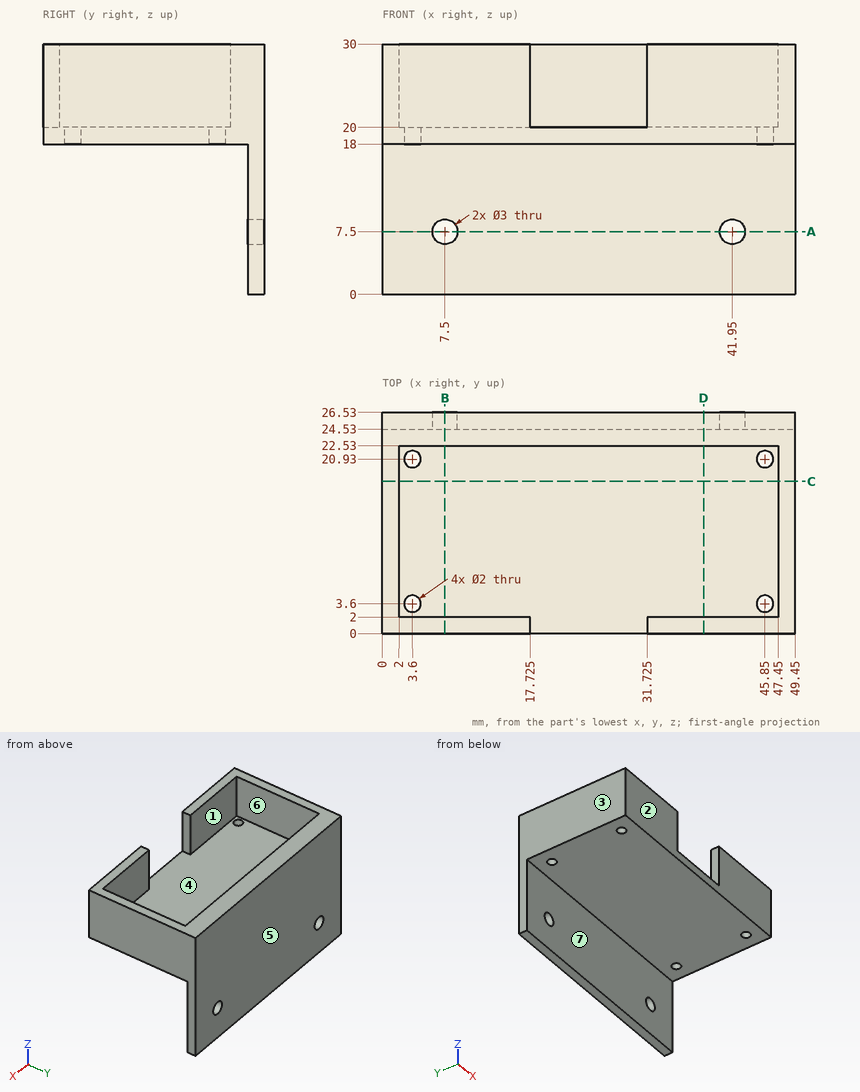
Could you check a few things on this drawing? It's one solid part, dimensions in mm from its lowest x, y, z. A direction names the side the tool comes from. Round coordinates to 2 decimals unless told otherwise and drop trailing zeros. Loops run counter-clockwise (first coordinate to the right, second up) from the corner with the lowest first, then second, coordinate; pieces in that order, holes last.
Q1. I want a section at D-D (x = 38.5). Write out the boundary of the cut face in (y, z).
Q2. On a 3-axis mill with a long thin cutter (end or side, diameter ignored), from which of +Z, -Z, +X, -X, +Y, -Y can I reach the whole of each face in a straight line? I mean the marked faces 5, 6 and 7. Say none if no direction works.
Q3. Please list where these lines run through material, in increasing order: L1, parallel to Y at x = 45.85, z = 18.5; L2, parallel to Y at x = 46, z = 25; L3, parallel to X at y = 14.5, z = 28.
Q4. I want a section at C-C (y = 18.25). Write out the boundary of the cut face in (x, z).
Q5. Thinking about a two-plate mould opening in X: for the marked faces 1, 2, 3 and 4, which applies, pulls with the +X half, pulls with the -X half, needs draft (parallel to the pull), parting line crosses it, or undercut?
Q6. I want a section at B-B (x = 7.5). Write out the boundary of the cut face in (y, z).
Q7. For P1, Ø9, axis at x = 14, z = 7.5, coming from the -Y side; P2, Ø5, axis at y = 15.5, z = 27.5, coming from the -X side; P3, Ø8, axis at x = 37.5, y = 11, coming from the +Z side, each with a flat end and sliding along its axis, tell me the tip position at first contact or that it passes through.
Q8. I want a section at A-A (z = 7.5). Write out the boundary of the cut face in (x, y), and give its area (3 significant figures).
Answer below:
1. outline: (0, 18) - (24.53, 18) - (24.53, 0) - (26.53, 0) - (26.53, 30) - (22.53, 30) - (22.53, 20) - (2, 20) - (2, 30) - (0, 30) - close
2. face 5: +Z, -Z, +X, -X, +Y
2. face 6: +Z
2. face 7: -Z, +X, -X, -Y
3. L1: y = 0 to 2.6, 4.6 to 19.93, 21.93 to 26.53
3. L2: y = 0 to 2, 22.53 to 26.53
3. L3: x = 0 to 2, 47.45 to 49.45
4. outline: (0, 18) - (49.45, 18) - (49.45, 30) - (47.45, 30) - (47.45, 20) - (2, 20) - (2, 30) - (0, 30) - close
5. face 1: undercut
5. face 2: needs draft
5. face 3: pulls with the -X half
5. face 4: undercut
6. outline: (0, 18) - (24.53, 18) - (24.53, 9) - (26.53, 9) - (26.53, 30) - (22.53, 30) - (22.53, 20) - (2, 20) - (2, 30) - (0, 30) - close; (24.53, 0) - (26.53, 0) - (26.53, 6) - (24.53, 6) - close
7. P1: stops at y = 24.53
7. P2: stops at x = 0
7. P3: stops at z = 20
8. outline: (0, 24.53) - (6, 24.53) - (6, 26.53) - (0, 26.53) - close; (9, 24.53) - (40.45, 24.53) - (40.45, 26.53) - (9, 26.53) - close; (43.45, 24.53) - (49.45, 24.53) - (49.45, 26.53) - (43.45, 26.53) - close
8. area: 86.9 mm2
